```python
from build123d import *

# Parameters (mm, degrees)
ESTRUSIONE_ESTRUSIONE1_DEPTH = 25
RACCORDO1_R                  = 2
TAGLIO_ESTRUSIONE1_DEPTH     = 29
TAGLIO_ESTRUSIONE3_DEPTH     = 38
SCHIZZO6_R                   = 4
SCHIZZO6_R_2                 = 1.5
TAGLIO_ESTRUSIONE4_DEPTH     = 38
SCHIZZO7_R                   = 4
SCHIZZO7_R_2                 = 1.5
TAGLIO_ESTRUSIONE5_DEPTH     = 29


with BuildPart() as part:
    # Schizzo1 → Estrusione-Estrusione1 (new body)
    with BuildSketch(Plane(origin=(0, 0, 0), x_dir=(1, 0, 0), z_dir=(0, 1, 0))):
        Polygon((11.035530567, -4.481060606), (-16.964469433, -4.481060606), (-16.964469433, 32.518939394), (-14.964469433, 32.518939394), (-14.964469433, -2.481060606), (11.035530567, -2.481060606), align=None)
    extrude(amount=ESTRUSIONE_ESTRUSIONE1_DEPTH)

    # Raccordo1
    raccordo1_edges = [part.edges().sort_by_distance(p)[0] for p in [
        (-16.964469433, 12.5, 4.481060606),
    ]]
    fillet(raccordo1_edges, radius=RACCORDO1_R)

    # Schizzo2 → Taglio-Estrusione1 (cut, through all)
    with BuildSketch(Plane.ZY.offset(16.964469433)):
        with BuildLine():
            ThreePointArc((-20.018939394, 0), (-28.857774159, 3.661165235), (-32.518939394, 12.5))
            Line((-32.518939394, 12.5), (-32.518939394, 0))
            Line((-32.518939394, 0), (-20.018939394, 0))
        make_face()
        with BuildLine():
            Line((-20.018939394, 25), (-32.518939394, 25))
            Line((-32.518939394, 25), (-32.518939394, 12.5))
            ThreePointArc((-32.518939394, 12.5), (-28.857774159, 21.338834765), (-20.018939394, 25))
        make_face()
    extrude(amount=-TAGLIO_ESTRUSIONE1_DEPTH, mode=Mode.SUBTRACT)

    # Schizzo4 → Taglio-Estrusione3 (cut, through all)
    with BuildSketch(Plane.XY.offset(4.481060606)):
        with BuildLine():
            Line((11.035530567, 25), (-1.964469433, 25))
            ThreePointArc((-1.964469433, 25), (7.052874966, 21.368038174), (11.035530567, 12.5))
            Line((11.035530567, 12.5), (11.035530567, 25))
        make_face()
        with BuildLine():
            Line((11.035530567, 0), (11.035530567, 11.554155381))
            ThreePointArc((11.035530567, 11.554155381), (7.676890272, 3.665306442), (-0.074234222, 0))
            Line((-0.074234222, 0), (11.035530567, 0))
        make_face()
    extrude(amount=-TAGLIO_ESTRUSIONE3_DEPTH, mode=Mode.SUBTRACT)

    # Schizzo6 → Taglio-Estrusione4 (cut, through all)
    with BuildSketch(Plane.XY.offset(4.481060606)):
        with Locations((-1.964469433, 12.5)):
            Circle(SCHIZZO6_R)
        with Locations((-1.964469433, 19.5)):
            Circle(SCHIZZO6_R_2)
        with Locations((-1.964469433, 5.5)):
            Circle(SCHIZZO6_R_2)
        with Locations((5.035530567, 12.5)):
            Circle(SCHIZZO6_R_2)
        with Locations((-8.964469433, 12.5)):
            Circle(SCHIZZO6_R_2)
    extrude(amount=-TAGLIO_ESTRUSIONE4_DEPTH, mode=Mode.SUBTRACT)

    # Schizzo7 → Taglio-Estrusione5 (cut, through all)
    with BuildSketch(Plane.ZY.offset(16.964469433)):
        with Locations((-20.018939394, 12.5)):
            Circle(SCHIZZO7_R)
        with Locations((-27.018939394, 12.5)):
            Circle(SCHIZZO7_R_2)
        with Locations((-20.018939394, 19.5)):
            Circle(SCHIZZO7_R_2)
        with Locations((-20.018939394, 5.5)):
            Circle(SCHIZZO7_R_2)
        with Locations((-13.018939394, 12.5)):
            Circle(SCHIZZO7_R_2)
    extrude(amount=-TAGLIO_ESTRUSIONE5_DEPTH, mode=Mode.SUBTRACT)


solid = part.part
```
Input: part model. Units: mm. Frame: model coordinates. A direction names the side the tool comes from. Give positions to 0.01 mm unless a question says otherwise; leave off trailing zeros. Order: outer loops, then holes, each group sorted by start corner. A loop starts at its lowest first (then second) coordinate and runs counter-clockwise, first axis right, second up. Notation, with made-up numbers: (-12, 58.5) - (40, 58.5) arc R23 ccw to (40, 97.5) - close; hole circle Ø3 at (2.25, -23.75). An arc over 180 degrees is marked (long way). One line per item, written item: value.
1. Cut plane C-C, the plane x = -4. Output: boundary loops of the cut face in (y, z).
Determined:
outline: (0, 2.48) - (9.06, 2.48) - (9.06, 4.48) - (0, 4.48) - close; (15.94, 2.48) - (25, 2.48) - (25, 4.48) - (15.94, 4.48) - close
2. Cut plane B-B, the plane z = -22.5. Output: boundary loops of the cut face in (x, y).
Determined:
outline: (-16.96, 0.25) - (-14.96, 0.25) - (-14.96, 9.36) - (-16.96, 9.36) - close; (-16.96, 15.64) - (-14.96, 15.64) - (-14.96, 24.75) - (-16.96, 24.75) - close
3. Cut plane A-A, the plane y = 19.5. Output: boundary loops of the cut face in (x, z), and give its area (3 significant figures).
Determined:
outline: (-16.96, -30.38) - (-14.96, -30.38) - (-14.96, -21.52) - (-16.96, -21.52) - close; (-16.96, -18.52) - (-14.96, -18.52) - (-14.96, 2.48) - (-3.46, 2.48) - (-3.46, 4.48) - (-14.96, 4.48) arc R2 ccw to (-16.96, 2.48) - close; (-0.46, 2.48) - (8.66, 2.48) - (8.66, 4.48) - (-0.46, 4.48) - close
area: 104 mm2
4. Line query: probe 1 along Z at (x, y) = (-11.75, 13); probe 2 along X at (y, z) = (6.5, -9). Output: solid intervals per line, ascending.
Determined:
probe 1: 2.48 to 4.48
probe 2: -16.96 to -14.96
5. Draft query along Y for faces 3 (the face through (-15.978, 12.676, -24.015)), 4 (the face through (-2, 21, 3)), 5 (the face through (7.76, 3.75, 3.5)), 6 (the face through (-16, 25, -5)). Return one class per face: released by +Y, released by -Y, zero draft, split by the parting line, or undercut.
Determined:
face 3: undercut
face 4: undercut
face 5: released by -Y
face 6: released by +Y
6. Reachability of faces 1 (the face through (-14.964, 12, -15)), 2 (the face through (-15.4, 0, -4.2)) from +Z, -Z, +X, -X, +Y, -Y: full face, straight path, thin tool, end or side. Return the list, or none.
Determined:
face 1: -Z, +X, +Y, -Y
face 2: +Z, -Z, +X, -X, -Y
7. Pin query (flat end, axial travel): pin 1 Ø3 at (x, y) = (-2, 6.5) entering from -Z; pin 2 Ø1 at (y, z) = (5, -6) entering from +X. Return the tip coordinate at first contact, or that it passes through.
Determined:
pin 1: z = 2.48
pin 2: x = -14.96
8. Cut plane D-D, the plane z = -4.5. Output: boundary loops of the cut face in (x, y), and give its area (3 significant figures).
Determined:
outline: (-16.96, 0) - (-14.96, 0) - (-14.96, 25) - (-16.96, 25) - close
area: 50.0 mm2
